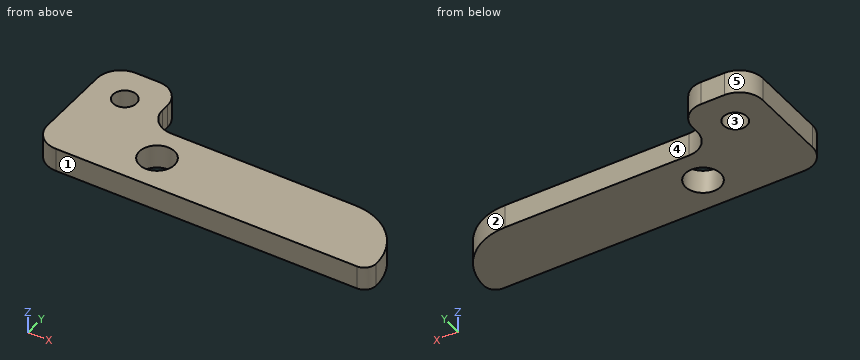
```python
from build123d import *

# Parameters (mm, degrees)
SKETCH1_R           = 1.5
SKETCH1_R_2         = 1
BOSS_EXTRUDE1_DEPTH = 2
FILLET7_R           = 5
FILLET8_R           = 1
FILLET9_R           = 2


with BuildPart() as part:
    # Sketch1 → Boss-Extrude1 (new body)
    with BuildSketch(Plane.XY):
        Polygon((-2.167750967, 169.712259216), (-2.167750967, 174.350350498), (-8.167750967, 174.350350498), (-8.167750967, 163.712259216), (0.596545219, 163.712259216), (20.559814769, 163.712259216), (20.559814769, 169.712259216), align=None)
        with Locations((0.559814769, 166.712259216)):
            Circle(SKETCH1_R, mode=Mode.SUBTRACT)
        with Locations((-5.167750967, 171.350350498)):
            Circle(SKETCH1_R_2, mode=Mode.SUBTRACT)
    extrude(amount=BOSS_EXTRUDE1_DEPTH)

    # Fillet7
    fillet7_edges = [part.edges().sort_by_distance(p)[0] for p in [
        (20.559814769, 169.712259216, 1),
    ]]
    fillet(fillet7_edges, radius=FILLET7_R)

    # Fillet8
    fillet8_edges = [part.edges().sort_by_distance(p)[0] for p in [
        (20.559814769, 163.712259216, 1),
    ]]
    fillet(fillet8_edges, radius=FILLET8_R - 0.0001)  # a hair under: the kernel refuses the full size

    # Fillet9
    fillet9_edges = [part.edges().sort_by_distance(p)[0] for p in [
        (-8.167750967, 174.350350498, 1),
        (-2.167750967, 174.350350498, 1),
        (-2.167750967, 169.712259216, 1),
        (-8.167750967, 163.712259216, 1),
    ]]
    fillet(fillet9_edges, radius=FILLET9_R)


solid = part.part
```
Check sheet for the modelled part. Datum: model origin and axes. Units: mm. Face numbers are marked on the shaded views. A direction names the side the tool comes from. Give positions to 0.01 mm unless a question says otherwise; leave off trailing zeros. Write each loop counter-clockwise with the first axis right and the second up, starting at its lowest first coordinate (ties: lowest second). Pieces come first, ordered by that corner, then holes.
Item 1: Cross-section at B-B (x = 0.25). Enter the section's corners in (y, z).
Item 2: Cross-section at D-D (x = 11.5). Enter the section's corners in (y, z).
Item 3: Scan lines: L1, parallel to Y at x = 3, z = 1.7; L2, parallel to Y at x = -4.5, z = 0.45; L3, parallel to X at y = 166.5, z = 1.05. Record each from-to range of solid material in increasing order.
Item 4: Gauge pin test, flat end, axial feed: pin 1 (0.7 mm diameter, centred on y = 172, z = 1.5, fed in from +X). Record the tip position at first contact, or that the pin passes through.
Item 5: Cross-section at A-A (y = 166). Enter the section's corners in (x, z).
Item 6: Cross-section at C-C (z = 1.55). Count the separate pieces of the cut face and the enclosed holes in it, and give its area (3 significant figures).
Item 7: Access from +Z, -Z, +X, -X, +Y, -Y to the whole of each face (thin tool, end or side, straight path). Record for the marked faces 4 and 5.
Item 8: Draft check along Y on the marked faces 1, 2 and 3. Enter one of: released by +Y, released by -Y, zero draft, split by the parting line, or undercut.
Report:
1. outline: (163.71, 0) - (165.24, 0) - (165.24, 2) - (163.71, 2) - close; (168.18, 0) - (169.71, 0) - (169.71, 2) - (168.18, 2) - close
2. outline: (163.71, 0) - (169.71, 0) - (169.71, 2) - (163.71, 2) - close
3. L1: y = 163.71 to 169.71
3. L2: y = 163.71 to 170.61, 172.09 to 174.35
3. L3: x = -8.17 to -0.93, 2.04 to 20.23
4. pin 1: stops at x = -2.17
5. outline: (-8.17, 0) - (-0.76, 0) - (-0.76, 2) - (-8.17, 2) - close; (1.88, 0) - (20.39, 0) - (20.39, 2) - (1.88, 2) - close
6. separate pieces: 1
6. enclosed holes: 2
6. area: 183 mm2
7. face 4: +Z, -Z, +X, +Y
7. face 5: +Z, -Z, -X, +Y
8. face 1: released by -Y
8. face 2: released by +Y
8. face 3: undercut
